Can you work these out from the model? Positions are in its coordinate system, mm. Face numbers are marked on the shaded views. A direction names the side the tool comes from. Round coordinates to 2 decimals unless told otherwise and drop trailing zeros. Write each loop counter-clockwise with the first axis right and the second up, starting at its lowest first coordinate (ties: lowest second). Pieces come first, ordered by that corner, then holes. Notation, with made-up numbers: M 7.5,14 L 38.5,14 A33 cw 38.5,49 Z; hole C -27.5,-18 d9. An arc over 180 degrees is marked long. Answer in a Markdown table with one row per item. Add a question column.
(1) If I drill on probe 1 along Y at (x, z) = (-3, -24.5); probe 2 along Z at (x, y) = (33, 24); probe 3 along Y at (x, z) = (-17, -5), over which ranges is the centre line in solid material (lowest first)?
(2) For the marked faces 1, 2 and 3, which set-ups out of +Z, -Z, +X, -X, +Y, -Y let a thin tool reach every point of the face, with its end or its side?
(3) I'm going to push flat-ended pins straight in: pin 1 (12 mm diameter, centred on y = -41, z = -33, fed in from +X); pin 2 (13.5 mm diameter, centred on y = 5.5, z = -22, fed in from +X); pin 3 (1.5 mm diameter, centred on x = 10, z = -29.5, fed in from -Y); pin 4 (6 mm diameter, centred on x = -22.5, z = -34.5, fed in from +Y). Where does each tip first touch, or does it pass through?
(4) Suppose I cut it at D-D, the plane z = -20. Write out the boundary of the cut face in (x, y), then the cut area to 3 significant figures.
(5) Suppose I cut it at C-C, the plane y = 17. Write out the boundary of the cut face in (x, z) (1 decimal), then the cut area to 3 significant figures.
(6) Suppose I cut it at A-A, the plane x = -16. Count the separate pieces of the cut face and the enclosed holes in it, then the cut area to 3 significant figures.
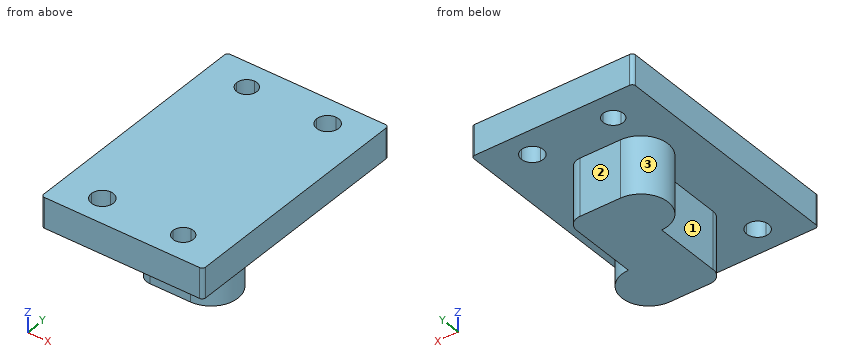
from build123d import *

# Parameters (mm, degrees)
F1_DEPTH = 41.275
F3_DEPTH = 14.2875
F5_DEPTH = 14.2875


with BuildPart() as f1:
    # F0 (on Top) → F1 (new body)
    with BuildSketch(Plane.XY):
        with BuildLine():
            Line((-6.3457395977, -31.7500010133), (12.7042604023, -31.7500010133))
            ThreePointArc((12.7042604023, -31.7500010133), (25.4042604023, -19.0500010133), (12.7042604023, -6.3500010133))
            Line((12.7042604023, -6.3500010133), (12.7042604023, 25.3999989867))
            ThreePointArc((12.7042604023, 25.3999989867), (10.8443884629, 29.8901270473), (6.3542604023, 31.7499989867))
            Line((6.3542604023, 31.7499989867), (-12.6957395977, 31.7499989867))
            ThreePointArc((-12.6957395977, 31.7499989867), (-25.3957395977, 19.0499989867), (-12.6957395977, 6.3499989867))
            Line((-12.6957395977, 6.3499989867), (-12.6957395977, -25.4000010133))
            ThreePointArc((-12.6957395977, -25.4000010133), (-10.8358676582, -29.8901290738), (-6.3457395977, -31.7500010133))
        make_face()
    extrude(amount=-F1_DEPTH)

    # F2 (on face) → F3 (join)
    with BuildSketch(Plane.XY):
        with BuildLine():
            Line((-36.5125, -57.15), (36.5125, -57.15))
            ThreePointArc((36.5125, -57.15), (37.6350320151, -56.6850320151), (38.1, -55.5625))
            Line((38.1, -55.5625), (38.1, 55.5625))
            ThreePointArc((38.1, 55.5625), (37.6350320151, 56.6850320151), (36.5125, 57.15))
            Line((36.5125, 57.15), (-36.5125, 57.15))
            ThreePointArc((-36.5125, 57.15), (-37.6350320151, 56.6850320151), (-38.1, 55.5625))
            Line((-38.1, 55.5625), (-38.1, -55.5625))
            ThreePointArc((-38.1, -55.5625), (-37.6350320151, -56.6850320151), (-36.5125, -57.15))
        make_face()
        with BuildLine():
            Line((-12.6957395977, 31.7499989867), (6.3542604023, 31.7499989867))
            ThreePointArc((6.3542604023, 31.7499989867), (10.8443884629, 29.8901270473), (12.7042604023, 25.3999989867))
            Line((12.7042604023, 25.3999989867), (12.7042604023, -6.3500010133))
            ThreePointArc((12.7042604023, -6.3500010133), (25.4042604023, -19.0500010133), (12.7042604023, -31.7500010133))
            Line((12.7042604023, -31.7500010133), (-6.3457395977, -31.7500010133))
            ThreePointArc((-6.3457395977, -31.7500010133), (-10.8358676582, -29.8901290738), (-12.6957395977, -25.4000010133))
            Line((-12.6957395977, -25.4000010133), (-12.6957395977, 6.3499989867))
            ThreePointArc((-12.6957395977, 6.3499989867), (-25.3957395977, 19.0499989867), (-12.6957395977, 31.7499989867))
        make_face(mode=Mode.SUBTRACT)
    extrude(amount=-F3_DEPTH)

    # F4 (on face) → F5 (cut)
    with BuildSketch(Plane.XY):
        with BuildLine():
            Line((19.05, 39.2938), (19.05, 44.45))
            Line((19.05, 44.45), (13.8938, 44.45))
            ThreePointArc((13.8938, 44.45), (15.4040160148, 40.8040160148), (19.05, 39.2938))
        make_face()
        with BuildLine():
            Line((19.05, 44.45), (24.2062, 44.45))
            ThreePointArc((24.2062, 44.45), (22.6959839852, 48.0959839852), (19.05, 49.6062))
            Line((19.05, 49.6062), (19.05, 44.45))
        make_face()
        with BuildLine():
            Line((19.05, 44.45), (19.05, 49.6062))
            ThreePointArc((19.05, 49.6062), (15.4040160148, 48.0959839852), (13.8938, 44.45))
            Line((13.8938, 44.45), (19.05, 44.45))
        make_face()
        with BuildLine():
            ThreePointArc((19.05, 39.2938), (22.6959839852, 40.8040160148), (24.2062, 44.45))
            Line((24.2062, 44.45), (19.05, 44.45))
            Line((19.05, 44.45), (19.05, 39.2938))
        make_face()
        with BuildLine():
            Line((-19.05, -44.45), (-13.8938, -44.45))
            ThreePointArc((-13.8938, -44.45), (-15.4040160148, -40.8040160148), (-19.05, -39.2938))
            Line((-19.05, -39.2938), (-19.05, -44.45))
        make_face()
        with BuildLine():
            ThreePointArc((-19.05, -49.6062), (-15.4040160148, -48.0959839852), (-13.8938, -44.45))
            Line((-13.8938, -44.45), (-19.05, -44.45))
            Line((-19.05, -44.45), (-19.05, -49.6062))
        make_face()
        with BuildLine():
            ThreePointArc((-24.2062, -44.45), (-22.6959839852, -48.0959839852), (-19.05, -49.6062))
            Line((-19.05, -49.6062), (-19.05, -44.45))
            Line((-19.05, -44.45), (-24.2062, -44.45))
        make_face()
        with BuildLine():
            Line((-24.2062, -44.45), (-19.05, -44.45))
            Line((-19.05, -44.45), (-19.05, -39.2938))
            ThreePointArc((-19.05, -39.2938), (-22.6959839852, -40.8040160148), (-24.2062, -44.45))
        make_face()
        with BuildLine():
            Line((-14.2875, 44.45), (-19.05, 44.45))
            Line((-19.05, 44.45), (-19.05, 39.6875))
            ThreePointArc((-19.05, 39.6875), (-15.6824039546, 41.0824039546), (-14.2875, 44.45))
        make_face()
        with BuildLine():
            ThreePointArc((-14.2875, 44.45), (-15.6824039546, 47.8175960454), (-19.05, 49.2125))
            Line((-19.05, 49.2125), (-19.05, 44.45))
            Line((-19.05, 44.45), (-14.2875, 44.45))
        make_face()
        with BuildLine():
            Line((-19.05, 44.45), (-19.05, 49.2125))
            ThreePointArc((-19.05, 49.2125), (-22.4175960454, 47.8175960454), (-23.8125, 44.45))
            Line((-23.8125, 44.45), (-19.05, 44.45))
        make_face()
        with BuildLine():
            Line((-19.05, 39.6875), (-19.05, 44.45))
            Line((-19.05, 44.45), (-23.8125, 44.45))
            ThreePointArc((-23.8125, 44.45), (-22.4175960454, 41.0824039546), (-19.05, 39.6875))
        make_face()
        with BuildLine():
            Line((19.05, -44.45), (23.8125, -44.45))
            ThreePointArc((23.8125, -44.45), (22.4175960454, -41.0824039546), (19.05, -39.6875))
            Line((19.05, -39.6875), (19.05, -44.45))
        make_face()
        with BuildLine():
            Line((14.2875, -44.45), (19.05, -44.45))
            Line((19.05, -44.45), (19.05, -39.6875))
            ThreePointArc((19.05, -39.6875), (15.6824039546, -41.0824039546), (14.2875, -44.45))
        make_face()
        with BuildLine():
            Line((19.05, -49.2125), (19.05, -44.45))
            Line((19.05, -44.45), (14.2875, -44.45))
            ThreePointArc((14.2875, -44.45), (15.6824039546, -47.8175960454), (19.05, -49.2125))
        make_face()
        with BuildLine():
            ThreePointArc((19.05, -49.2125), (22.4175960454, -47.8175960454), (23.8125, -44.45))
            Line((23.8125, -44.45), (19.05, -44.45))
            Line((19.05, -44.45), (19.05, -49.2125))
        make_face()
    extrude(amount=-F5_DEPTH, mode=Mode.SUBTRACT)


solid = f1.part
Calculated:
| question | item | result |
|---|---|---|
| 1 | probe 1 | -31.75 to 31.75 |
| 1 | probe 2 | -14.29 to 0 |
| 1 | probe 3 | -57.15 to -49.18, -39.72 to 40.15, 48.75 to 57.15 |
| 2 | face 1 | -Z, -X, -Y |
| 2 | face 2 | -Z, +X, -X, +Y |
| 2 | face 3 | -Z, -X |
| 3 | pin 1 | through |
| 3 | pin 2 | x = 12.7 |
| 3 | pin 3 | y = -31.75 |
| 3 | pin 4 | y = 29.77 |
| 4 | outline | M -12.7,-25.4 A6.35 ccw -6.35,-31.75 L 12.7,-31.75 A12.7 ccw 12.7,-6.35 L 12.7,25.4 A6.35 ccw 6.35,31.75 L -12.7,31.75 A12.7 ccw -12.7,6.35 Z |
| 4 | area | 2,100 mm² |
| 5 | outline | M -38.1,-14.3 L -25.2,-14.3 L -25.2,-41.3 L 12.7,-41.3 L 12.7,-14.3 L 38.1,-14.3 L 38.1,0 L -38.1,0 Z |
| 5 | area | 2,110 mm² |
| 6 | separate pieces | 3 |
| 6 | enclosed holes | 0 |
| 6 | area | 2,070 mm² |
